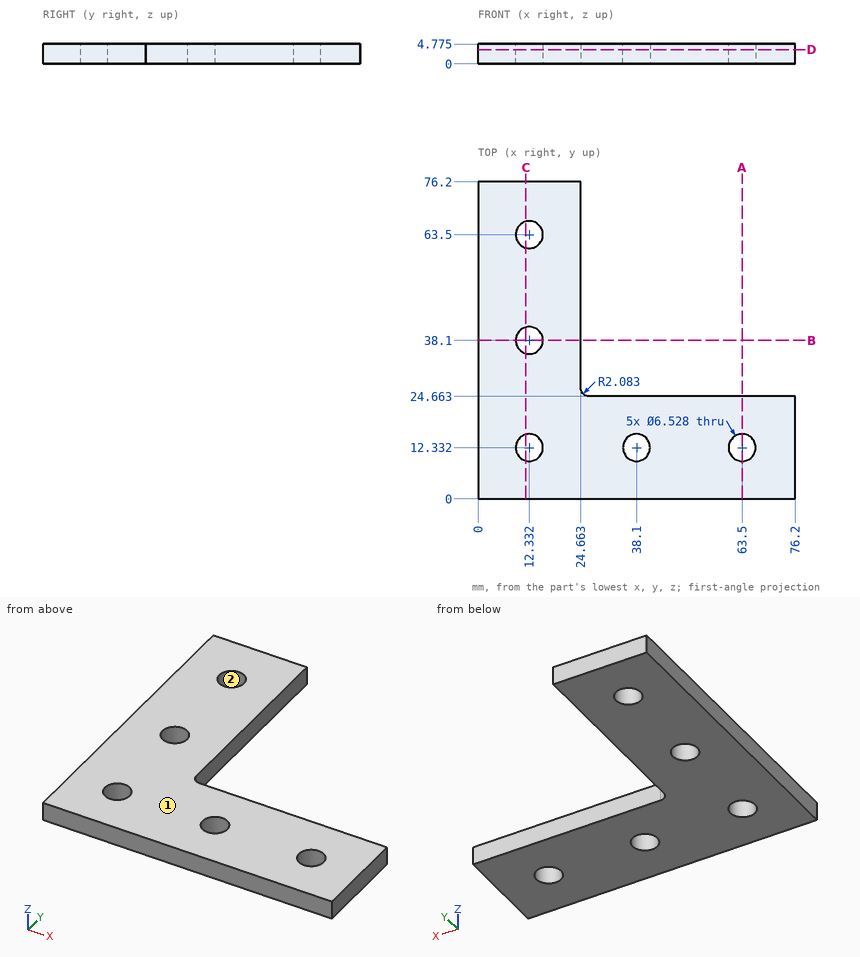
Can you work these out from the drawing? Everything is in mm from the part's minimum corner. Give positions to 0.01 mm unless a question says otherwise; leave off trailing zeros. Order: outer loops, then holes, each group sorted by start corner. A loop starts at its lowest first (then second) coordinate and runs counter-clockwise, first axis right, second up. Notation, with made-up numbers: M 58,31.25 L 64,31.25 A17 ccw 64,36.25 Z; hole C 76,-33.5 d6. An arc over 180 degrees is marked long. Use a Markdown table: item, result. Add a question column.
1. If we mould it in two halves opening along Y, with no side actions, what happens to the marked faces 1 and 2? For each: +Y half, -Y half, draft (parallel to the pull), parting line (faces both ways), or undercut.
2. I need wall thicknesses on probe 1 along Y at (x, z) = (38, 1.4); probe 2 along Y at (x, z) = (10.5, 4) (1 decimal); probe 3 along Y at (x, z) = (13, 1.05) (1 decimal). Which ranges of each line are inside material? Lowest first, please. Write a range as from..to.
3. Suppose I cut it at A-A (x = 63.5). List the corners of the cut face in (y, z) for me (1 decimal), and give its area (3 significant figures).
4. Suppose I cut it at C-C (x = 11.5). List the corners of the cut face in (y, z) for me (1 decimal).
5. Suppose I cut it at D-D (z = 3.4). List the corners of the cut face in (x, y) for me (1 decimal).
6. For pin 1 Ø2.5 at (y, z) = (39, 3) entering from +X; pin 2 Ø1 at (x, z) = (55.5, 3) entering from +Y, each with a flat end and sliding along its axis, tell me the tip position at first contact or that it passes through.
Results list:
| question | item | result |
|---|---|---|
| 1 | face 1 | draft |
| 1 | face 2 | undercut |
| 2 | probe 1 | y = 0..9.07, 15.59..24.66 |
| 2 | probe 2 | y = 0..9.6, 15..35.4, 40.8..60.8, 66.2..76.2 |
| 2 | probe 3 | y = 0..9.1, 15.5..34.9, 41.3..60.3, 66.7..76.2 |
| 3 | outline | M 0,0 L 9.1,0 L 9.1,4.8 L 0,4.8 Z; M 15.6,0 L 24.7,0 L 24.7,4.8 L 15.6,4.8 Z |
| 3 | area | 86.6 mm² |
| 4 | outline | M 0,0 L 9.2,0 L 9.2,4.8 L 0,4.8 Z; M 15.5,0 L 34.9,0 L 34.9,4.8 L 15.5,4.8 Z; M 41.3,0 L 60.3,0 L 60.3,4.8 L 41.3,4.8 Z; M 66.7,0 L 76.2,0 L 76.2,4.8 L 66.7,4.8 Z |
| 5 | outline | M 0,0 L 76.2,0 L 76.2,24.7 L 26.7,24.7 A2.1 cw 24.7,26.7 L 24.7,76.2 L 0,76.2 Z; hole C 12.3,12.3 d6.5; hole C 12.3,38.1 d6.5; hole C 12.3,63.5 d6.5; hole C 38.1,12.3 d6.5; hole C 63.5,12.3 d6.5 |
| 6 | pin 1 | stops at x = 24.66 |
| 6 | pin 2 | stops at y = 24.66 |
